```python
from build123d import *

# Parameters (mm, degrees)
F0_W     = 508
F0_H     = 508
F1_DEPTH = 12.7
F2_W     = 482.6
F2_H     = 482.6
F3_DEPTH = 150
F4_W     = 102
F4_H     = 62
F5_DEPTH = 50.8


with BuildPart() as f1:
    # F0 (on Top) → F1 (new body)
    with BuildSketch(Plane.XY):
        Rectangle(F0_W, F0_H)
    extrude(amount=-F1_DEPTH)

    # F2 (on face) → F3 (join)
    with BuildSketch(Plane.XY):
        Polygon((-241.3, 254), (-254, 254), (-254, 241.3), (-254, -233.078346), (-254, -241.3), (-254, -254), (-241.3, -254), (241.3, -254), (254, -254), (254, -241.3), (254, 241.3), (254, 254), (241.3, 254), align=None)
        Rectangle(F2_W, F2_H, mode=Mode.SUBTRACT)
    extrude(amount=F3_DEPTH)

    # F4 (on face) → F5 (cut)
    with BuildSketch(Plane.XZ.offset(254)):
        with Locations((0.197696, 84.359624)):
            Rectangle(F4_W, F4_H)
    extrude(amount=-F5_DEPTH, mode=Mode.SUBTRACT)


solid = f1.part
```
Geometry: final body of the model. Coordinates: model frame, mm. A direction names the side the tool comes from. Coordinates: 2 decimals unless noted, no trailing zeros. Order: outer loops, then holes, each group sorted by start corner. A loop starts at its lowest first (then second) coordinate and runs counter-clockwise, first axis right, second up. Notation, with made-up numbers: (75.25, 3) - (105.25, 3) arc R10 ccw to (105.25, 11) - close; hole circle Ø5 at (79, -36). An arc over 180 degrees is marked (long way). Write each question's results on one line, items separated by ' | '.
1) Section C-C, the plane z = 77. Return loops of the section in (x, y), plus the area to 3 significant figures.
Results list:
outline: (-254, -254) - (-50.8, -254) - (-50.8, -241.3) - (-241.3, -241.3) - (-241.3, 241.3) - (241.3, 241.3) - (241.3, -241.3) - (51.2, -241.3) - (51.2, -254) - (254, -254) - (254, 254) - (-254, 254) - close | area: 23,900 mm^2
2) Pin query (flat end, axial travel): pin 1 (8 mm diameter, centred on x = 162, y = 102, fed in from +Z). Return the tip coordinate at first contact, or that it passes through.
Results list:
pin 1: z = 0
3) Section B-B, the plane x = 157.5. Return loops of the section in (y, z).
Results list:
outline: (-254, -12.7) - (254, -12.7) - (254, 150) - (241.3, 150) - (241.3, 0) - (-241.3, 0) - (-241.3, 150) - (-254, 150) - close
4) Section A-A, the plane z = 129.5. Return loops of the section in (x, y).
Results list:
outline: (-254, -254) - (254, -254) - (254, 254) - (-254, 254) - close; hole (-241.3, -241.3) - (241.3, -241.3) - (241.3, 241.3) - (-241.3, 241.3) - close
5) Set-up query: faces 5 (the flat face through (241.3, -3, 74)), 6 (the flat face through (51.198, -248, 84)), 7 (the flat face through (254, -4, 68)). Return all of +Z, -Z, +X, -X, +Y, -Y with unobstructed straight access to the full face (end or side cutting, diameter ignored); none if empty.
Results list:
face 5: +Z | face 6: -Y | face 7: +Z, -Z, +X, +Y, -Y
6) Pull-direction query (Y, two-part tool) for faces 1 (the flat face through (-50.802, -248, 84)), 2 (the flat face through (4, 254, 68)), 3 (the flat face through (-4, -254, 49)), 4 (the flat face through (-241.3, -3, 74)); classes: pulls with the +Y half, pulls with the -Y half, needs draft (parallel to the pull), parting line crosses it, or undercut.
Results list:
face 1: needs draft | face 2: pulls with the +Y half | face 3: pulls with the -Y half | face 4: undercut
7) Line query: line 1 (Y direction, x = -75, z = 49.5); line 2 (Z direction, x = 152.5, y = -173). Output: solid intervals per line, ascending. Write a range as from..to.
Results list:
line 1: -254..-241.3, 241.3..254 | line 2: -12.7..0
